from build123d import *

# Parameters (mm, degrees)
SKETCH_1_W      = 24
SKETCH_1_H      = 130
SKETCH_1_R      = 1.5
SKETCH_1_R_2    = 4.5
EXTRUDE_1_DEPTH = 1.5


with BuildPart() as part:
    # 草图1 → 凸台-拉伸1 (new body)
    with BuildSketch(Plane.XY):
        Rectangle(SKETCH_1_W, SKETCH_1_H)
        with Locations((0, 15)):
            Circle(SKETCH_1_R, mode=Mode.SUBTRACT)
        with Locations((0, -55)):
            Circle(SKETCH_1_R, mode=Mode.SUBTRACT)
        with Locations(Location((0, 55, 0), (0, 0, 180))):
            Circle(SKETCH_1_R, mode=Mode.SUBTRACT)
        with Locations((0, -15)):
            Circle(SKETCH_1_R_2, mode=Mode.SUBTRACT)
        with BuildLine():
            Line((-7.4, -1.8), (-7.4, 0.2))
            ThreePointArc((-7.4, 0.2), (-5, 2.6), (-2.6, 0.2))
            Line((-2.6, 0.2), (-2.6, -1.8))
            ThreePointArc((-2.6, -1.8), (-5, -4.2), (-7.4, -1.8))
        make_face(mode=Mode.SUBTRACT)
        with BuildLine():
            Line((7.4, -1.8), (7.4, 0.2))
            ThreePointArc((7.4, 0.2), (5, 2.6), (2.6, 0.2))
            Line((2.6, 0.2), (2.6, -1.8))
            ThreePointArc((2.6, -1.8), (5, -4.2), (7.4, -1.8))
        make_face(mode=Mode.SUBTRACT)
        with BuildLine():
            Line((-7.4, -48.2), (-7.4, -50.2))
            ThreePointArc((-7.4, -50.2), (-5, -52.6), (-2.6, -50.2))
            Line((-2.6, -50.2), (-2.6, -48.2))
            ThreePointArc((-2.6, -48.2), (-5, -45.8), (-7.4, -48.2))
        make_face(mode=Mode.SUBTRACT)
        with BuildLine():
            Line((7.4, -48.2), (7.4, -50.2))
            ThreePointArc((7.4, -50.2), (5, -52.6), (2.6, -50.2))
            Line((2.6, -50.2), (2.6, -48.2))
            ThreePointArc((2.6, -48.2), (5, -45.8), (7.4, -48.2))
        make_face(mode=Mode.SUBTRACT)
    extrude(amount=EXTRUDE_1_DEPTH)


solid = part.part
Check sheet for the modelled part. Datum: model origin and axes. Units: mm. A direction names the side the tool comes from. Round coordinates to 2 decimals unless told otherwise and drop trailing zeros. Loops run counter-clockwise (first coordinate to the right, second up) from the corner with the lowest first, then second, coordinate; pieces in that order, holes last. Notation, with made-up numbers: M 36,53.5 L 64,53.5 A4 cw 64,59.5 Z; hole C -37,13.25 d2. An arc over 180 degrees is marked long. One line per item, written item: value.
(1) Release check for a two-part mould opening along X. For faces 3 (the face through (0, 1, 0)), 4 (the face through (-1.11, 16.01, 0.74)) record: +X half, -X half, draft (parallel to the pull), parting line (faces both ways), or undercut.
Computed values:
face 3: draft
face 4: undercut
(2) Sectioned sample at C-C, the plane x = 0. Record the cut outline in (y, z).
Computed values:
outline: M -65,0 L -56.5,0 L -56.5,1.5 L -65,1.5 Z; M -53.5,0 L -19.5,0 L -19.5,1.5 L -53.5,1.5 Z; M -10.5,0 L 13.5,0 L 13.5,1.5 L -10.5,1.5 Z; M 16.5,0 L 53.5,0 L 53.5,1.5 L 16.5,1.5 Z; M 56.5,0 L 65,0 L 65,1.5 L 56.5,1.5 Z
(3) Depth check by flat-ended pin: pin 1 Ø2.5 at (x, y) = (0, 15) entering from -Z. Enter the tip coordinate at first touch or a pass-through.
Computed values:
pin 1: passes through
(4) Sectioned sample at B-B, the plane z = 0.35. Count the separate pieces of the cut face and the enclosed holes in it, then the cut area to 3 significant figures.
Computed values:
separate pieces: 1
enclosed holes: 8
area: 2,920 mm^2
(5) Access from +Z, -Z, +X, -X, +Y, -Y to the whole of each face (thin tool, end or side, straight path). Record for faces 1 (the face through (0, 1, 1.5)), 2 (the face through (-5.05, -52.6, 0.74)).
Computed values:
face 1: +Z, +X, -X, +Y, -Y
face 2: +Z, -Z
(6) Sectioned sample at A-A, the plane y = -55. Record the cut outline in (x, z).
Computed values:
outline: M -12,0 L -1.5,0 L -1.5,1.5 L -12,1.5 Z; M 1.5,0 L 12,0 L 12,1.5 L 1.5,1.5 Z
(7) Thickness scan on line 1 (Y direction, x = 0, z = 0.5); line 2 (X direction, y = -49, z = 0.8); line 3 (Y direction, x = -6.5, z = 1). Record the ranges inside material, lowest first.
Computed values:
line 1: y = -65 to -56.5, -53.5 to -19.5, -10.5 to 13.5, 16.5 to 53.5, 56.5 to 65
line 2: x = -12 to -7.4, -2.6 to 2.6, 7.4 to 12
line 3: y = -65 to -52.07, -46.33 to -3.67, 2.07 to 65
(8) Sectioned sample at D-D, the plane x = -6. Record the cut outline in (y, z).
Computed values:
outline: M -65,0 L -52.38,0 L -52.38,1.5 L -65,1.5 Z; M -46.02,0 L -3.98,0 L -3.98,1.5 L -46.02,1.5 Z; M 2.38,0 L 65,0 L 65,1.5 L 2.38,1.5 Z
